Part model, mm, in its own coordinate system. A direction names the side the tool comes from. Round coordinates to 2 decimals unless told otherwise and drop trailing zeros. Order: outer loops, then holes, each group sorted by start corner. A loop starts at its lowest first (then second) coordinate and runs counter-clockwise, first axis right, second up. Notation, with made-up numbers: (17, 41) - (32, 41) arc R24 cw to (32, 69) - close; hole circle Ø11 at (-37.5, 88.25). An arc over 180 degrees is marked (long way). Answer as a JSON object with one key per item and string values.
```python
from build123d import *

# Parameters (mm, degrees)
F0_R     = 3.2385
F1_DEPTH = 6.35


with BuildPart() as f1:
    # F0 (on Front) → F1 (new body)
    with BuildSketch(Plane.XZ):
        with BuildLine():
            Line((19.016519, 18.216161), (-2.098458, 18.216161))
            ThreePointArc((-2.098458, 18.216161), (-3.26134, 18.436786), (-4.262609, 19.068))
            Line((-4.262609, 19.068), (-18.587252, 32.412178))
            Line((-18.587252, 32.412178), (-19.245879, 33.025725))
            ThreePointArc((-19.245879, 33.025725), (-28.353882, 34.24271), (-33.345191, 26.527555))
            Line((-33.345191, 26.527555), (-28.95716, 5.867742))
            ThreePointArc((-28.95716, 5.867742), (-28.905248, 5.539737), (-28.887881, 5.208104))
            Line((-28.887881, 5.208104), (-28.887881, -7.133039))
            Line((-28.887881, -7.133039), (22.191519, -7.133039))
            Line((22.191519, -7.133039), (22.191519, 15.041161))
            ThreePointArc((22.191519, 15.041161), (21.261583, 17.286225), (19.016519, 18.216161))
        make_face()
        with Locations((-24.760381, 26.445761)):
            Circle(F0_R, mode=Mode.SUBTRACT)
        with BuildLine():
            Line((-19.245879, 33.025725), (-18.587252, 32.412178))
            ThreePointArc((-18.587252, 32.412178), (-18.908519, 32.72759), (-19.245879, 33.025725))
        make_face()
    extrude(amount=F1_DEPTH)


solid = f1.part
```
Item 1: Tool access for faces 1 (the flat face through (-31.18, -3.13, 16.34)), 2 (the flat face through (9, -3, 18.216)): list every direction of +Z, -Z, +X, -X, +Y, -Y with a clear straight run to the whole face (end or side of a thin tool).
Taken from the geometry:
{"face 1": "-Z, -X, +Y, -Y", "face 2": "+Z, +X, +Y, -Y"}
Item 2: Cut at C-C (x = 1). Write the cut outline in (y, z).
Taken from the geometry:
{"outline": "(-6.35, -7.13) - (0, -7.13) - (0, 18.22) - (-6.35, 18.22) - close"}
Item 3: Two-plate mould, pull along X, no slides. Class faces 3 (the flat face through (-28.888, -3, -1)), 4 (the cylindrical face through (21.29, -3.13, 17.26)), 5 (the flat face through (-6, 0, 10)), 6 (the cylindrical face through (-23.019, -3.131, 29.176)): pulls with the +X half, pulls with the -X half, needs draft (parallel to the pull), parting line crosses it, or undercut.
Taken from the geometry:
{"face 3": "pulls with the -X half", "face 4": "pulls with the +X half", "face 5": "needs draft", "face 6": "undercut"}
Item 4: Probe L1, parallel to Z at x = 15.5, y = -5; L2, parallel to X at y = -3.75, z = 2; L3, parallel to Z at x = -26.5, y = -5. List the from-to ranges inside material, lowest first. Write a range as from..to.
Taken from the geometry:
{"L1": "-7.13..18.22", "L2": "-28.89..22.19", "L3": "-7.13..23.71, 29.18..34.85"}
Item 5: Drop flat-ended pins along their axis: P1, Ø2, axis at x = 13.5, y = -4, coming from the +Z side; P2, Ø1.5, axis at y = -1, z = 15, coming from the -X side; P3, Ø2, axis at y = -5, z = 27, coming from the +X side; P4, Ø4, axis at x = -15, z = 26.5, coming from the +Y side. Give the stop position or say it passes through.
Taken from the geometry:
{"P1": "z = 18.22", "P2": "x = -31.06", "P3": "x = -11.7", "P4": "y = 0"}
Item 6: Cut at B-B (z = -1.5). Write the cut outline in (x, y).
Taken from the geometry:
{"outline": "(-28.89, -6.35) - (22.19, -6.35) - (22.19, 0) - (-28.89, 0) - close"}
